The model under review builds one solid part; all positions refer to its coordinate system, in mm. Round coordinates to 2 decimals unless told otherwise and drop trailing zeros. Write each loop counter-clockwise with the first axis right and the second up, starting at its lowest first coordinate (ties: lowest second). Pieces come first, ordered by that corner, then holes. Notation, with made-up numbers: M 63,11.5 L 97,11.5 A22 cw 97,28.5 Z; hole C 60.5,86.5 d10. An arc over 180 degrees is marked long. Write item = value, one per line. Start each with the question number.
Item 1: To check wall thickness, follow line 1 along Y through (x, z) = (10, 1.4); line 2 along Y through (x, z) = (-26, 1.5); line 3 along X through (y, z) = (-8.5, 1.35). State the ranges of each line that lie inside material, in increasing order.
Item 2: Take a section at D-D, the plane x = -35.5. Give the boundary of the cut face in (y, z), plus the area to 3 significant figures.
Item 3: For pin 1 Ø4.5 at (x, y) = (10, 10) entering from +Z, flat-tipped, find the tip position at first contact; note if it passes through.
Item 4: Take a section at B-B, the plane z = 1.45. Give the number of separate pieces and of enclosed holes in the cut face, plus the area to 3 significant figures.
Item 5: Take a section at C-C, the plane y = 14. Give the boundary of the cut face in (x, z), plus the area to 3 significant figures.
Item 6: Take a section at A-A, the plane x = 26. Give the boundary of the cut face in (y, z), plus the area to 3 significant figures.
from build123d import *

# Parameters (mm, degrees)
SKETCH_1_W      = 100
SKETCH_1_H      = 36.5
SKETCH_1_R      = 5.5
SKETCH_1_R_2    = 2.5
EXTRUDE_1_DEPTH = 2


with BuildPart() as part:
    # Эскиз1 → Вытянуть1 (new body)
    with BuildSketch(Plane.XY):
        Rectangle(SKETCH_1_W, SKETCH_1_H)
        with Locations((35.5, 0)):
            Circle(SKETCH_1_R, mode=Mode.SUBTRACT)
        with Locations(Location((-35.5, 0, 0), (0, 0, 180))):
            Circle(SKETCH_1_R, mode=Mode.SUBTRACT)
        with Locations((-41, 10)):
            Circle(SKETCH_1_R_2, mode=Mode.SUBTRACT)
        with Locations((-26, 12.5)):
            Circle(SKETCH_1_R_2, mode=Mode.SUBTRACT)
        with Locations((-10, 10)):
            Circle(SKETCH_1_R_2, mode=Mode.SUBTRACT)
        with Locations(Location((-10, -10, 0), (0, 0, 180))):
            Circle(SKETCH_1_R_2, mode=Mode.SUBTRACT)
        with Locations(Location((-26, -12.5, 0), (0, 0, 180))):
            Circle(SKETCH_1_R_2, mode=Mode.SUBTRACT)
        with Locations(Location((-41, -10, 0), (0, 0, 180))):
            Circle(SKETCH_1_R_2, mode=Mode.SUBTRACT)
        with Locations(Location((10, 10, 0), (0, 0, 180))):
            Circle(SKETCH_1_R_2, mode=Mode.SUBTRACT)
        with Locations((10, -10)):
            Circle(SKETCH_1_R_2, mode=Mode.SUBTRACT)
        with Locations((26, -12.5)):
            Circle(SKETCH_1_R_2, mode=Mode.SUBTRACT)
        with Locations(Location((26, 12.5, 0), (0, 0, 180))):
            Circle(SKETCH_1_R_2, mode=Mode.SUBTRACT)
        with Locations(Location((41, 10, 0), (0, 0, 180))):
            Circle(SKETCH_1_R_2, mode=Mode.SUBTRACT)
        with Locations((41, -10)):
            Circle(SKETCH_1_R_2, mode=Mode.SUBTRACT)
    extrude(amount=EXTRUDE_1_DEPTH)


solid = part.part
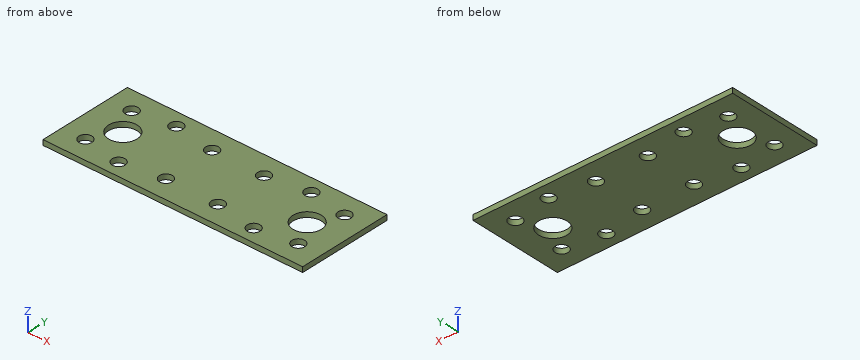
Response values:
q1.line_1 = -18.25 to -12.5, -7.5 to 7.5, 12.5 to 18.25
q1.line_2 = -18.25 to -15, -10 to 10, 15 to 18.25
q1.line_3 = -50 to -43, -39 to -12, -8 to 8, 12 to 39, 43 to 50
q2.outline = M -18.25,0 L -5.5,0 L -5.5,2 L -18.25,2 Z; M 5.5,0 L 18.25,0 L 18.25,2 L 5.5,2 Z
q2.area = 51.0 mm2
q3.pin_1 = through
q4.separate_pieces = 1
q4.enclosed_holes = 14
q4.area = 3,220 mm2
q5.outline = M -50,0 L -28,0 L -28,2 L -50,2 Z; M -24,0 L 24,0 L 24,2 L -24,2 Z; M 28,0 L 50,0 L 50,2 L 28,2 Z
q5.area = 184 mm2
q6.outline = M -18.25,0 L -15,0 L -15,2 L -18.25,2 Z; M -10,0 L 10,0 L 10,2 L -10,2 Z; M 15,0 L 18.25,0 L 18.25,2 L 15,2 Z
q6.area = 53.0 mm2
